CAD build for the part. Positions are in the model's coordinates, mm. Face numbers are marked on the shaded views. A direction names the side the tool comes from. Coordinates: 2 decimals unless noted, no trailing zeros. Order: outer loops, then holes, each group sorted by start corner. A loop starts at its lowest first (then second) coordinate and runs counter-clockwise, first axis right, second up. Notation, with made-up numbers: (81, -2.75) -> (110, -2.75) arc R20 ccw to (110, 15.25) -> close; hole circle Ø11 at (74.5, 48). An arc over 180 degrees is marked (long way). Use one line per item in the form item = value. Start each with the question number.
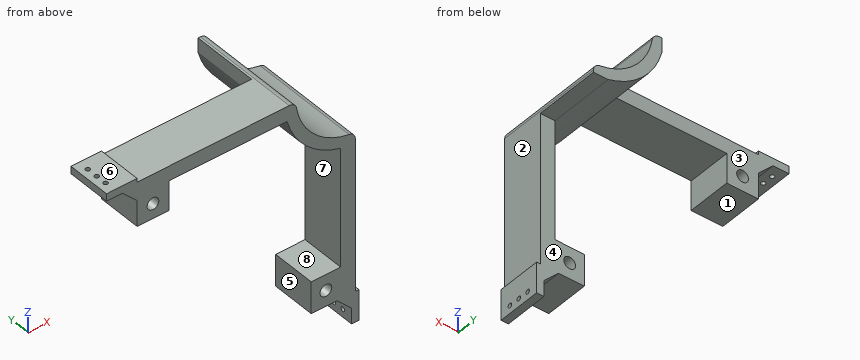
from build123d import *

# Parameters (mm, degrees)
SKETCH2_R           = 4
BOSS_EXTRUDE1_DEPTH = 30
SKETCH10_R          = 1.5
CUT_EXTRUDE1_DEPTH  = 10
SKETCH11_R          = 1.5
CUT_EXTRUDE3_DEPTH  = 10
BOSS_EXTRUDE2_DEPTH = 45


with BuildPart() as part:
    # Sketch2 → Boss-Extrude1 (new body)
    with BuildSketch(Plane(origin=(0, 0, 0), x_dir=(1, 0, 0), z_dir=(0, 1, 0))):
        with BuildLine():
            Line((-2.5, 47.410441888), (-2.5, 49.444413233))
            Line((-2.5, 49.444413233), (-2.5, 151))
            Line((-2.5, 151), (0, 151))
            Line((0, 151), (0, 171.795711314))
            Line((0, 171.795711314), (-5, 171.795711314))
            Line((-5, 171.795711314), (-5, 161))
            Line((-5, 161), (-15, 151))
            Line((-15, 151), (-32.5, 151))
            Line((-32.5, 151), (-32.5, 129.444413233))
            Line((-32.5, 129.444413233), (-12.5, 129.444413233))
            Line((-12.5, 129.444413233), (-12.5, 48.928519291))
            ThreePointArc((-12.5, 48.928519291), (-35.70889245, 35.70889245), (-48.928519291, 12.5))
            Line((-48.928519291, 12.5), (-129.444413233, 12.5))
            Line((-129.444413233, 12.5), (-129.444413233, 32.5))
            Line((-129.444413233, 32.5), (-151, 32.5))
            Line((-151, 32.5), (-151, 15))
            Line((-151, 15), (-161, 5))
            Line((-161, 5), (-171.795711314, 5))
            Line((-171.795711314, 5), (-171.795711314, 0))
            Line((-171.795711314, 0), (-151, 0))
            Line((-151, 0), (-151, 2.5))
            Line((-151, 2.5), (-49.444413233, 2.5))
            Line((-49.444413233, 2.5), (-47.410441888, 2.5))
            ThreePointArc((-47.410441888, 2.5), (-44.162846624, 3.698273419), (-42.471854191, 6.71875))
            ThreePointArc((-42.471854191, 6.71875), (-30.405591591, 30.405591591), (-6.71875, 42.471854191))
            ThreePointArc((-6.71875, 42.471854191), (-3.698273419, 44.162846624), (-2.5, 47.410441888))
        make_face()
        with Locations(Location((-22.5, 140.222206617, 0), (0, 0, 270))):
            Circle(SKETCH2_R, mode=Mode.SUBTRACT)
        with Locations(Location((-140.222206617, 22.5, 0), (0, 0, 270))):
            Circle(SKETCH2_R, mode=Mode.SUBTRACT)
    extrude(amount=BOSS_EXTRUDE1_DEPTH)

    # Sketch10 → Cut-Extrude1 (cut)
    with BuildSketch(Plane.ZY.offset(5)):
        with Locations((-166.397855657, 22.5)):
            Circle(SKETCH10_R)
        with Locations((-166.397855657, 15)):
            Circle(SKETCH10_R)
        with Locations((-166.397855657, 7.5)):
            Circle(SKETCH10_R)
    extrude(amount=-CUT_EXTRUDE1_DEPTH, mode=Mode.SUBTRACT)

    # Sketch11 → Cut-Extrude3 (cut)
    with BuildSketch(Plane(origin=(0, 0, -5), x_dir=(-1, 0, 0), z_dir=(0, 0, -1))):
        with Locations((166.397855657, 22.5)):
            Circle(SKETCH11_R)
        with Locations((166.397855657, 15)):
            Circle(SKETCH11_R)
        with Locations((166.397855657, 7.5)):
            Circle(SKETCH11_R)
    extrude(amount=-CUT_EXTRUDE3_DEPTH, mode=Mode.SUBTRACT)

    # Sketch13 → Boss-Extrude2 (add)
    with BuildSketch(Plane(origin=(0, 30, 0), x_dir=(1, 0, 0), z_dir=(0, 1, 0))):
        with BuildLine():
            Line((-48.928519291, 12.5), (-48.928519291, 2.5))
            Line((-48.928519291, 2.5), (-47.410441888, 2.5))
            ThreePointArc((-47.410441888, 2.5), (-44.162846624, 3.698273419), (-42.471854191, 6.71875))
            ThreePointArc((-42.471854191, 6.71875), (-30.405591591, 30.405591591), (-6.71875, 42.471854191))
            ThreePointArc((-6.71875, 42.471854191), (-3.698273419, 44.162846624), (-2.5, 47.410441888))
            Line((-2.5, 47.410441888), (-2.5, 48.928519291))
            Line((-2.5, 48.928519291), (-12.5, 48.928519291))
            ThreePointArc((-12.5, 48.928519291), (-35.70889245, 35.70889245), (-48.928519291, 12.5))
        make_face()
    extrude(amount=BOSS_EXTRUDE2_DEPTH)


solid = part.part
1) Cut at D-D on z = -94. Give the cut face in (x, y).
2) Drop flat-ended pins along their axis: P1, Ø3.5, axis at x = -166.4, y = 7.5, coming from the +Z side; P2, Ø16, axis at x = -134.5, z = -15, coming from the +Y side; P3, Ø2.5, axis at x = -166.4, y = 15, coming from the +Z side; P4, Ø3, axis at x = -9.5, y = 52, coming from the -Z side. Give the stop position or say it passes through.
3) 3-axis set-ups, long thin cutter, end or side, ignore diameter. For the marked faces 1, 2, 3 and 4: which of +Z, -Z, +X, -X, +Y, -Y reach the whole face in a straight line?
4) Probe L1, parallel to Z at x = -140.5, y = 5; L2, parallel to Z at x = -23.5, y = 13; L3, parallel to X at y = 12, z = -21.5. List the from-to ranges inside material, lowest first.
5) Cut at B-B on y = 40.5. Give the cut face in (x, z), then the cut area to 3 significant figures.
6) Cut at A-A on x = -22.5. Give the cut face in (y, z), then the cut area to 3 significant figures.
7) Cut at C-C on z = -22.5. Give the cut face in (x, y).
8) Two-plate mould, pull along Z, no slides. Class the marked faces 5, 6, 7 and 8: released by +Z, released by -Z, zero draft, split by the parting line, or undercut.
Values follow:
q1.outline = (-12.5, 0) -> (-2.5, 0) -> (-2.5, 30) -> (-12.5, 30) -> close
q2.P1 = 0
q2.P2 = 30
q2.P3 = through
q2.P4 = -48.93
q3.face_1 = -Z, -X, +Y, -Y
q3.face_2 = +Z, +X, +Y, -Y
q3.face_3 = +Z, -Z, -X, +Y
q3.face_4 = -Z, +X, -X, +Y
q4.L1 = -32.5 to -26.49, -18.51 to -2.5
q4.L2 = -151 to -144.1, -136.35 to -129.44, -44.7 to -36.01
q4.L3 = -151 to -144.1, -136.35 to -129.44, -45.69 to -37.24
q5.outline = (-48.93, -12.5) arc R50.5 ccw to (-12.5, -48.93) -> (-2.5, -48.93) -> (-2.5, -47.41) arc R5 ccw to (-6.72, -42.47) arc R43 cw to (-42.47, -6.72) arc R5 ccw to (-47.41, -2.5) -> (-48.93, -2.5) -> close
q5.area = 487 mm^2
q6.outline = (0, -151) -> (30, -151) -> (30, -144.22) -> (0, -144.22) -> close; (0, -136.22) -> (30, -136.22) -> (30, -129.44) -> (0, -129.44) -> close; (0, -45.21) -> (75, -45.21) -> (75, -36.64) -> (0, -36.64) -> close
q6.area = 1,050 mm^2
q7.outline = (-151, 0) -> (-144.22, 0) -> (-144.22, 30) -> (-151, 30) -> close; (-136.22, 0) -> (-129.44, 0) -> (-129.44, 30) -> (-136.22, 30) -> close; (-45.21, 0) -> (-36.64, 0) -> (-36.64, 75) -> (-45.21, 75) -> close
q8.face_5 = zero draft
q8.face_6 = released by +Z
q8.face_7 = undercut
q8.face_8 = undercut
